For this review, use the dimensioned drawing (mm, ordinates from the lowest corner) and the shaded views. Give positions to 0.01 mm unless a question says otherwise; leave off trailing zeros. Order: outer loops, then holes, each group sorted by start corner. A loop starts at its lowest first (then second) coordinate and runs counter-clockwise, first axis right, second up. Notation, with made-up numbers: M 68,49.25 L 77,49.25 A35 ccw 77,83.25 Z; hole C 18,8 d2. An arc over 180 degrees is marked long. One line per question, with ' | ' between items. Start each with the question number.
1. The part is to be moulded in two halves that separate along Z. For the marked faces 1, 2 and 3, say which applies: +Z half, -Z half, draft (parallel to the pull), parting line (faces both ways), or undercut.
2. We need section A-A on x = 19.05. Write out the cut boundary in (y, z) (1 decimal).
3. We need section B-B on z = 45. Count the separate pieces of the cut face and the enclosed holes in it, then the cut area to 3 significant figures.
4. Wall thickness on L1, parallel to X at y = 6.35, z = 7.5; L2, parallel to Y at x = 9, z = 5; L3, parallel to Z at x = 3.55, y = 6.35: over which ranges is each line inside the solid? List them lowest first.
5. Insertion check: P1, Ø4, axis at x = 8.89, y = 6.35, coming from the +Z side; P2, Ø1.5, axis at y = 2.5, z = 38, coming from the -X side; P3, Ø4.5, axis at x = 29.21, y = 6.35, coming from the +Z side; P4, Ø4, axis at x = 29.21, y = 6.35, coming from the -Z side. Each pin has a flat end and moves straight along its axis. Give the tip position at first contact, or say it passes through.
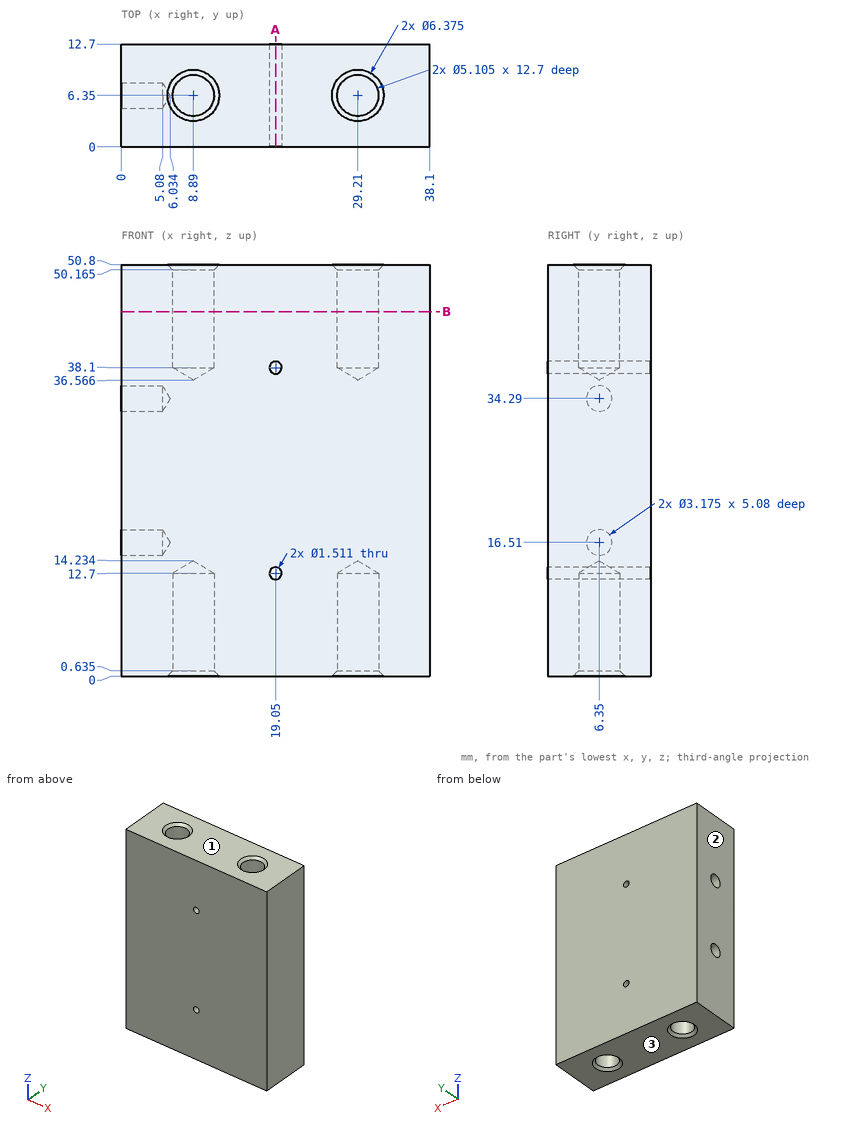
Entries:
1) face 1: +Z half | face 2: draft | face 3: -Z half
2) outline: M 0,0 L 12.7,0 L 12.7,11.9 L 0,11.9 Z; M 0,13.5 L 12.7,13.5 L 12.7,37.3 L 0,37.3 Z; M 0,38.9 L 12.7,38.9 L 12.7,50.8 L 0,50.8 Z
3) separate pieces: 1 | enclosed holes: 2 | area: 443 mm^2
4) L1: x = 0 to 6.34, 11.44 to 26.66, 31.76 to 38.1 | L2: y = 0 to 3.8, 8.9 to 12.7 | L3: z = 0 to 14.92, 18.1 to 32.7, 35.88 to 50.8
5) P1: stops at z = 37.77 | P2: stops at x = 0 | P3: stops at z = 37.92 | P4: stops at z = 13.03
